Autodesk Inventor part; units mm, degrees
ref_plane "YZ Plane" through (0, 0, 0) normal (1, 0, 0) x (0, 1, 0)
ref_plane "XZ Plane" through (0, 0, 0) normal (0, 1, 0) x (-1, 0, 0)
ref_plane "XY Plane" through (0, 0, 0) normal (0, 0, 1) x (1, 0, 0)
sketch "スケッチ1" plane through (0, 0, 0) normal (0, 0, 1) x (1, 0, 0)
  line L0 (-12.5, 25) -> (12.5, 25)
  line L1 (12.5, 25) -> (12.5, -25)
  line L2 (12.5, -25) -> (-12.5, -25)
  line L3 (-12.5, -25) -> (-12.5, 25)
  line L4 (-10.5, 23) -> (10.5, 23)
  line L5 (10.5, 23) -> (10.5, -23)
  line L6 (10.5, -23) -> (-10.5, -23)
  line L7 (-10.5, -23) -> (-10.5, 23)
  point P0 (0, 0)
  dimension "d0" = 25
  dimension "d1" = 50
  dimension "d2" = 46
  dimension "d3" = 21
  dimension "d4" = 25
  dimension "d5" = 23
  dimension "d6" = 10.5
  dimension "d7" = 12.5
extrude "押し出し1" add sketch "スケッチ1" along normal blind 60
sketch "スケッチ2" plane through (-12.5, 25, 0) normal (0, 1, 0) x (1, 0, 0)
  line L0 (0, 0) -> (25, 0)
  line L1 (0, 0) -> (0, -60)
  arc A0 (6, -33.5) -> (19, -33.5) centre (12.5, -33.5) ccw
  line L2 (6, -33.5) -> (6, 0)
  line L3 (19, -33.5) -> (19, 0)
  point P0 (12.5, 0)
  dimension "d10" = 13
  dimension "d11" = 33.5
  dimension "d12" = 12.5
extrude "押し出し2" cut sketch "スケッチ2" against normal blind 2
sketch "スケッチ3" plane through (-12.5, 25, 60) normal (0, 1, 0) x (1, 0, 0)
  arc A0 (6, 26.5) -> (19, 26.5) centre (12.5, 26.5) ccw
  circle A1 centre (4.5, 20) radius 1
  circle A2 centre (4.5, 56) radius 1
  circle A3 centre (20.5, 56) radius 1
  circle A4 centre (20.5, 20) radius 1
  point P0 (12.5, 60)
  dimension "d15" = 6.5
  dimension "d16" = 6.5
  dimension "d17" = 2
  dimension "d18" = 8
  dimension "d19" = 8
  dimension "d20" = 8
  dimension "d21" = 8
  dimension "d22" = 29.5
  dimension "d23" = 29.5
hole "穴1" at (-8, 25, 4) at (8, 25, 4) at (8, 25, 40) at (-8, 25, 40) direction (0, -1, 0) diameter 2 depth 2 tip angle 118 counterbore diameter 4 counterbore depth 0.5
sketch "スケッチ4" plane through (-12.5, -25, 0) normal (0, -1, 0) x (1, 0, 0)
  line L0 (25, 0) -> (0, 0)
  line L1 (25, 0) -> (25, 60)
  circle A0 centre (12.5, 10.5) radius 2
  point P0 (12.5, 0)
  dimension "d31" = 4
  dimension "d32" = 12.5
  dimension "d33" = 10.5
hole "穴2" at (0, -25, 10.5) direction (0, 1, 0) diameter 4 end through all
sketch "スケッチ5" plane through (-12.5, 25, 60) normal (0, 1, 0) x (1, 0, 0)
  arc A0 (6, 26.5) -> (19, 26.5) centre (12.5, 26.5) ccw
  circle A1 centre (20.5, 4) radius 1.5
  circle A2 centre (4.5, 4) radius 1.5
  circle A3 centre (20.5, 20) radius 2
  circle A4 centre (4.5, 20) radius 2
  point P0 (12.5, 60)
  dimension "d46" = 8
  dimension "d47" = 8
  dimension "d57" = 3
  dimension "d120" = 16
  dimension "d121" = 16
hole "穴4" at (-8, 25, 56) at (8, 25, 56) direction (0, -1, 0) diameter 3 end through all
thread "ねじ1"
thread "ねじ2"
thread "ねじ3"
thread "ねじ4"
sketch "スケッチ7" plane through (-12.5, -25, 0) normal (0, -1, 0) x (1, 0, 0)
  line L0 (25, 0) -> (25, 60)
  circle A0 centre (12.5, 30) radius 4
  circle A1 centre (4.5, 56) radius 1.5
  circle A2 centre (12.5, 10.5) radius 2
  point P0 (12.5, 0)
  dimension "d79" = 8
  dimension "d80" = 12.5
  dimension "d118" = 19.5
  dimension "d119" = 26
hole "穴5" at (0, -25, 30) direction (0, 1, 0) diameter 8 end through all
sketch "スケッチ8" plane through (12.5, -25, 0) normal (1, 0, 0) x (0, 0, -1)
  line L0 (-60, 50) -> (-60, 0)
  line L1 (0, 0) -> (-60, 0)
  circle A0 centre (-45, 33) radius 1.5
  circle A1 centre (-45, 17) radius 1.5
  circle A2 centre (-55, 40) radius 1.5
  circle A3 centre (-55, 10) radius 1.5
  line L2 (0, 50) -> (-60, 50)
  line L3 (0, 50) -> (0, 0)
  point P0 (0, 25)
  dimension "d88" = 16
  dimension "d90" = 3
  dimension "d91" = 15
  dimension "d93" = 17
  dimension "d101" = 30
  dimension "d113" = 10
  dimension "d114" = 15
  dimension "d115" = 5
  dimension "d116" = 5
  dimension "d117" = 60
hole "穴7" at (12.5, 8, 45) at (12.5, -8, 45) at (12.5, -15, 55) at (12.5, 15, 55) direction (-1, 0, 0) diameter 3 end through all
properties part number "07" material "アルミニウム 6061"
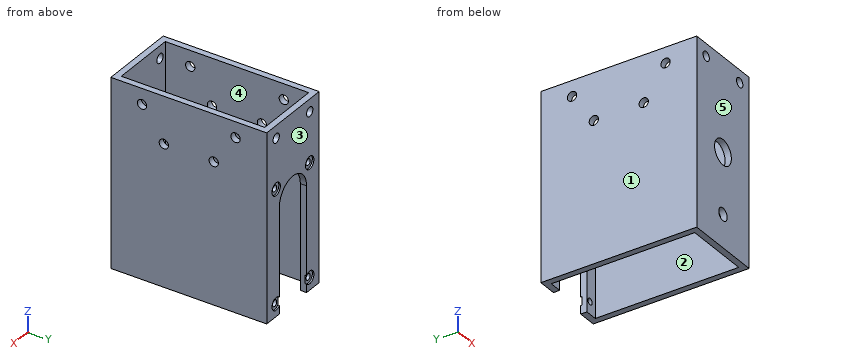
Geometry check sheet. Reference: the model listing, model coordinates, mm. Face numbers are marked on the shaded views. A direction names the side the tool comes from. Give positions to 0.01 mm unless a question says otherwise; leave off trailing zeros. Write each loop counter-clockwise with the first axis right and the second up, starting at its lowest first coordinate (ties: lowest second). Pieces come first, ordered by that corner, then holes. Notation, with made-up numbers: (-25.75, -15.75) - (9.25, -15.75) arc R20 ccw to (9.25, 15.25) - close; hole circle Ø10 at (56, 49.25). An arc over 180 degrees is marked (long way). Put each result on its own line as item: value.
1. Go/stop test with a flat-tipped pin: pin 1 (1.2 mm diameter, centred on x = 8.5, z = 39.5, fed in from +Y). Record where the tip stops, or that it passes through.
Ans:
pin 1: stops at y = 24.5
2. Sectioned sample at A-A, the plane x = 0. Enter the section's corners in (y, z).
Ans:
outline: (-25, 0) - (-23, 0) - (-23, 8.5) - (-25, 8.5) - close; (-25, 12.5) - (-23, 12.5) - (-23, 26) - (-25, 26) - close; (-25, 34) - (-23, 34) - (-23, 60) - (-25, 60) - close; (23, 40) - (25, 40) - (25, 60) - (23, 60) - close
3. Sectioned sample at D-D, the plane z = 45. Enter the section's corners in (x, y).
Ans:
outline: (-12.5, -25) - (12.5, -25) - (12.5, -9.5) - (10.5, -9.5) - (10.5, -23) - (-10.5, -23) - (-10.5, -9.5) - (-12.5, -9.5) - close; (-12.5, -6.5) - (-10.5, -6.5) - (-10.5, 6.5) - (-12.5, 6.5) - close; (-12.5, 9.5) - (-10.5, 9.5) - (-10.5, 23) - (10.5, 23) - (10.5, 9.5) - (12.5, 9.5) - (12.5, 25) - (-12.5, 25) - close; (10.5, -6.5) - (12.5, -6.5) - (12.5, 6.5) - (10.5, 6.5) - close
4. Sectioned sample at B-B, the plane y = -2.5. Enter the section's corners in (x, z).
Ans:
outline: (-12.5, 0) - (-10.5, 0) - (-10.5, 60) - (-12.5, 60) - close; (10.5, 0) - (12.5, 0) - (12.5, 60) - (10.5, 60) - close
5. Sectioned sample at C-C, the plane z = 30. Enter the section's corners in (x, y).
Ans:
outline: (-12.5, -25) - (-4, -25) - (-4, -23) - (-10.5, -23) - (-10.5, 23) - (-6.5, 23) - (-6.5, 25) - (-12.5, 25) - close; (4, -25) - (12.5, -25) - (12.5, 25) - (6.5, 25) - (6.5, 23) - (10.5, 23) - (10.5, -23) - (4, -23) - close
6. Thickness scan on line 1 (Y direction, x = -11.75, z = 45); line 2 (Z direction, x = -8, y = 24.85); line 3 (Z direction, x = 8, y = 23.95). Record the ranges inside material, lowest first.
Ans:
line 1: y = -25 to -9.5, -6.5 to 6.5, 9.5 to 25
line 2: z = 0 to 2, 6 to 38, 42 to 54.5, 57.5 to 60
line 3: z = 0 to 3, 5 to 39, 41 to 54.5, 57.5 to 60
7. Draft check along X on the marked faces 1, 2 and 3. Enter one of: +X half, -X half, draft (parallel to the pull), parting line (faces both ways), or undercut.
Ans:
face 1: -X half
face 2: undercut
face 3: draft
8. Set-up check for the marked faces 4 and 5: record each of +Z, -Z, +X, -X, +Y, -Y from which the full face is reachable in a straight line by a thin tool's end or side.
Ans:
face 4: +Z, -Z
face 5: +Z, -Z, +X, -X, -Y
